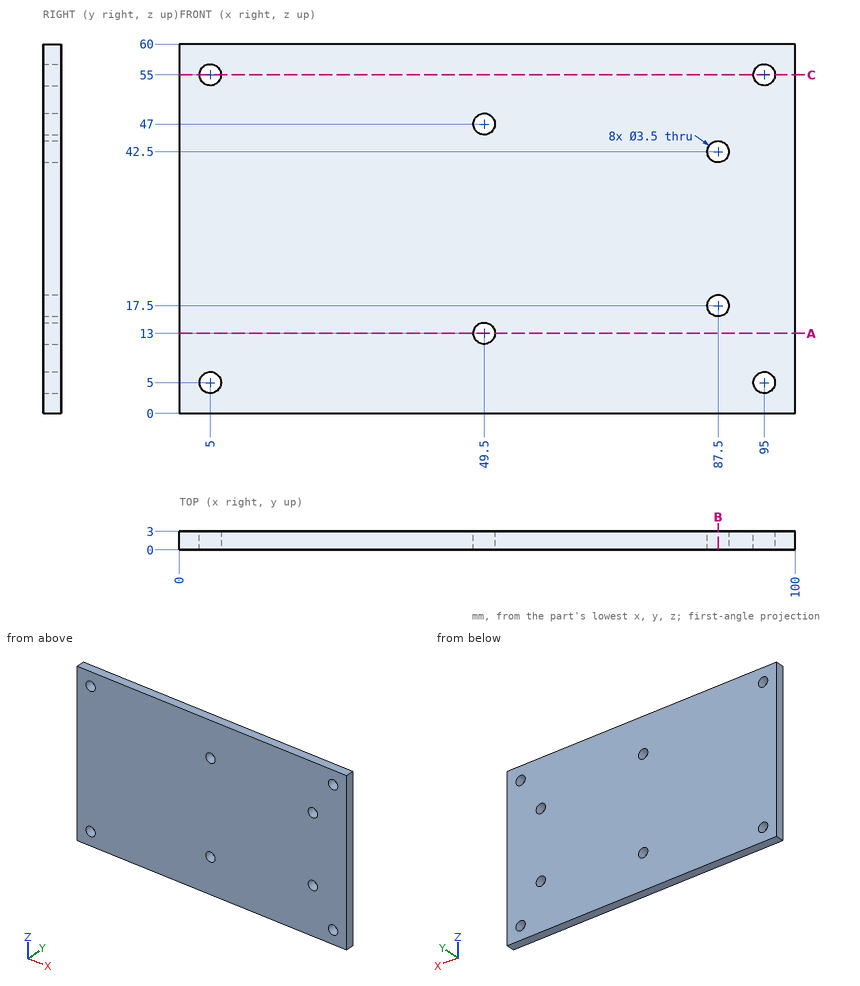
Design review of the part shown in the three views and the two pictorial views. Dimensions are in mm from the part's minimum x, y and z. Give positions to 0.01 mm unless a question says otherwise; leave off trailing zeros. Loops run counter-clockwise (first coordinate to the right, second up) from the corner with the lowest first, then second, coordinate; pieces in that order, holes last. Notation, with made-up numbers: (60.5, 24.5) -> (108.5, 24.5) arc R30 cw to (108.5, 48.5) -> close; hole circle Ø11 at (-35, 17). An arc over 180 degrees is marked (long way). Answer as a JSON object with one key per item and string values. Group by question number.
Q1. Wall thickness on line 1 along Z through (x, y) = (95, 2.3); line 2 along X through (y, z) = (2.05, 5); line 3 along Z through (x, y) = (87.5, 1.8): over which ranges is each line inside the solid? List them lowest first.
Q2. Take a section at B-B (x = 87.5). Write out the cut boundary in (y, z).
Q3. Insertion check: pin 1 (4.5 mm diameter, centred on x = 95, z = 55, fed in from -Y); pin 2 (3 mm diameter, centred on x = 87.5, z = 42.5, fed in from -Y). Each pin has a flat end and moves straight along its axis. Give the tip position at first contact, or say it passes through.
Q4. Take a section at A-A (z = 13). Write out the cut boundary in (x, y).
Q5. Take a section at C-C (z = 55). Write out the cut boundary in (x, y), plus the area to 3 significant figures.
Answer below:
{
 "1": {"line 1": "z = 0 to 3.25, 6.75 to 53.25, 56.75 to 60", "line 2": "x = 0 to 3.25, 6.75 to 93.25, 96.75 to 100", "line 3": "z = 0 to 15.75, 19.25 to 40.75, 44.25 to 60"},
 "2": {"outline": "(0, 0) -> (3, 0) -> (3, 15.75) -> (0, 15.75) -> close; (0, 19.25) -> (3, 19.25) -> (3, 40.75) -> (0, 40.75) -> close; (0, 44.25) -> (3, 44.25) -> (3, 60) -> (0, 60) -> close"},
 "3": {"pin 1": "stops at y = 0", "pin 2": "passes through"},
 "4": {"outline": "(0, 0) -> (47.75, 0) -> (47.75, 3) -> (0, 3) -> close; (51.25, 0) -> (100, 0) -> (100, 3) -> (51.25, 3) -> close"},
 "5": {"outline": "(0, 0) -> (3.25, 0) -> (3.25, 3) -> (0, 3) -> close; (6.75, 0) -> (93.25, 0) -> (93.25, 3) -> (6.75, 3) -> close; (96.75, 0) -> (100, 0) -> (100, 3) -> (96.75, 3) -> close", "area": "279 mm2"}
}
